Check sheet for the drawn part. Datum: minimum x, y, z corner. Units: mm. Give positions to 0.01 mm unless a question says otherwise; leave off trailing zeros. Order: outer loops, then holes, each group sorted by start corner. A loop starts at its lowest first (then second) coordinate and runs counter-clockwise, first axis right, second up.
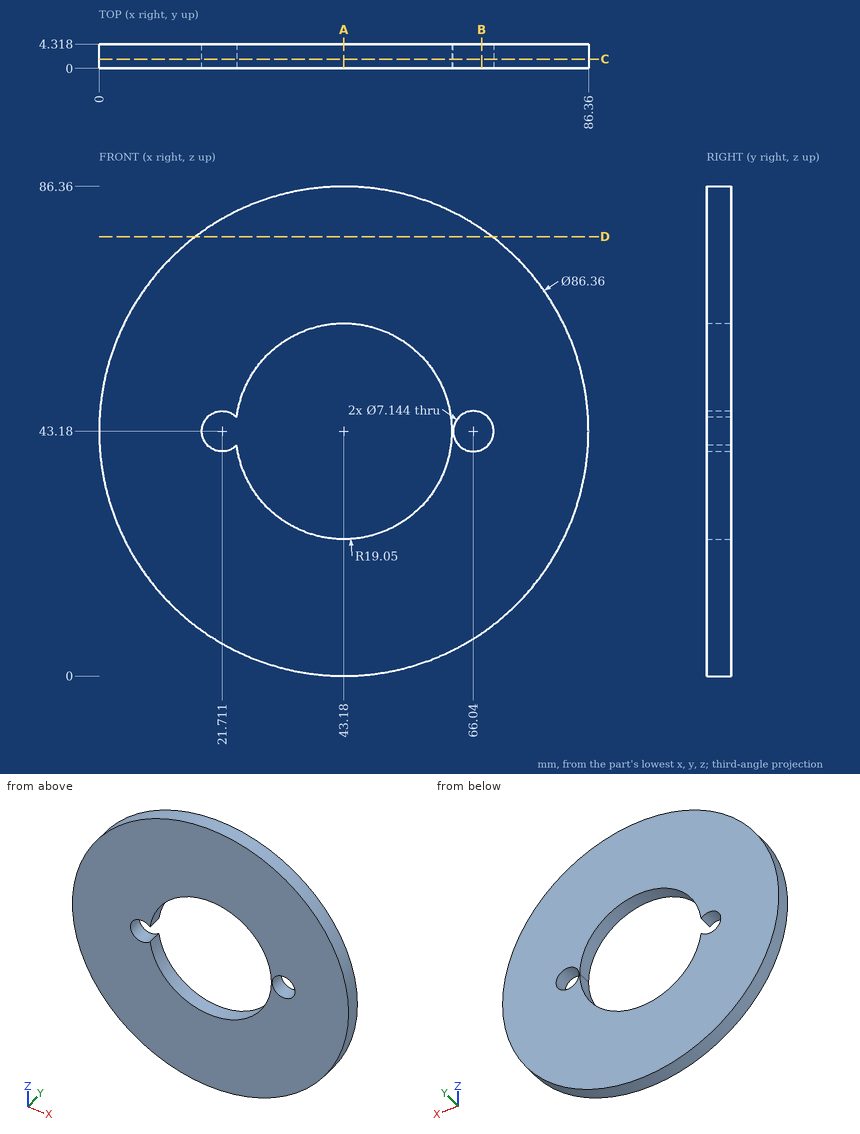
(1) Go/stop test with flat-tipped pins: pin 1 (10 mm diameter, centred on x = 29.5, z = 22.5, fed in from -Y); pin 2 (1 mm diameter, centred on x = 43.5, y = 2, fed in from +Z); pin 3 (1 mm diameter, centred on y = 2, z = 15, fed in from +X). Record where each tip stops, or that it passes through.
Solved:
pin 1: stops at y = 0
pin 2: stops at z = 86.36
pin 3: stops at x = 76.32
(2) Scan lines: line 1 (X direction, y = 3.8, z = 40) (1 decimal); line 2 (Z direction, x = 51.5, y = 2.5); line 3 (Z direction, x = 21, y = 0.65). Record each from-to range of solid material in increasing order.
Solved:
line 1: x = 0.1 to 20.1, 23.3 to 24.4, 62 to 64.4, 67.7 to 86.2
line 2: z = 0.81 to 26.04, 60.32 to 85.55
line 3: z = 6.13 to 39.68, 46.68 to 80.23
(3) Section check D-D, the plane z = 77.5. Enter the section's corners in (x, y).
Solved:
outline: (16.98, 0) - (69.38, 0) - (69.38, 4.32) - (16.98, 4.32) - close
(4) Section check B-B, the plane x = 67.5. Enter the section's corners in (y, z).
Solved:
outline: (0, 7.5) - (4.32, 7.5) - (4.32, 39.92) - (0, 39.92) - close; (0, 46.44) - (4.32, 46.44) - (4.32, 78.86) - (0, 78.86) - close
(5) Section check A-A, the plane x = 43.18. Enter the section's corners in (y, z), then the cut area to 3 significant figures.
Solved:
outline: (0, 0) - (4.32, 0) - (4.32, 24.13) - (0, 24.13) - close; (0, 62.23) - (4.32, 62.23) - (4.32, 86.36) - (0, 86.36) - close
area: 208 mm2
(6) Section check C-C, the plane y = 1.65. Enter the section's corners in (x, z), then the cut area to 3 significant figures.
Solved:
outline: circle Ø86.36 at (43.18, 43.18); hole (24.29, 40.71) arc R19.05 ccw (long way) to (24.29, 45.65) arc R3.57 ccw (long way) to start; hole circle Ø7.14 at (66.04, 43.18)
area: 4,640 mm2
